```python
from build123d import *

# Parameters (mm, degrees)
F0_W     = 10
F0_H     = 40
F1_DEPTH = 180
F2_R     = 7
F3_DEPTH = 10.001
F4_W     = 40
F4_H     = 40
F4_R     = 7
F5_DEPTH = 10


with BuildPart() as f1:
    # F0 (on Right) → F1 (new body)
    with BuildSketch(Plane.YZ):
        Rectangle(F0_W, F0_H)
    extrude(amount=-F1_DEPTH)

    # F2 (on face) → F3 (cut, through all)
    with BuildSketch(Plane.XZ.offset(5)):
        with Locations((-160, 0)):
            Circle(F2_R)
        with Locations((-20, 0)):
            Circle(F2_R)
    extrude(amount=-F3_DEPTH, mode=Mode.SUBTRACT)

    # F4 (on face) → F5 (join)
    with BuildSketch(Plane.XZ.offset(5)):
        with Locations((-20, 0)):
            Rectangle(F4_W, F4_H)
        with Locations((-20, 0)):
            Circle(F4_R, mode=Mode.SUBTRACT)
    extrude(amount=F5_DEPTH)


solid = f1.part
```
Check sheet for the modelled part. Datum: model origin and axes. Units: mm. A direction names the side the tool comes from. Coordinates: 2 decimals unless noted, no trailing zeros. Loops run counter-clockwise (first coordinate to the right, second up) from the corner with the lowest first, then second, coordinate; pieces in that order, holes last.
1) Access from +Z, -Z, +X, -X, +Y, -Y to the whole of each face (thin tool, end or side, straight path). Record for faces 1 (the face through (-40, -10, 0)), 2 (the face through (-89, 5, 0)).
2) Gauge pin test, flat ends, axial feed: pin 1 (12 mm diameter, centred on x = -142.5, z = 2.5, fed in from -Y); pin 2 (1.5 mm diameter, centred on x = -88, y = -7, fed in from +Z); pin 3 (8 mm diameter, centred on y = -11.5, z = 0, fed in from -X). Record the tip position at first contact, or that the pin passes through.
3) Sectioned sample at C-C (y = -1). Record the boundary of the cut face in (x, z), and give its area (3 significant figures).
4) Sectioned sample at A-A (x = -160). Record the boundary of the cut face in (y, z).
5) Material ranges on probe 1 along X at (y, z) = (-1.5, -0.5); probe 2 along Z at (x, y) = (-20, -3); probe 3 along X at (y, z) = (-1.5, -5), recorded low to high.
6) Release check for a two-part mould opening along Z. For faces 3 (the face through (-71, -3, 20)), 4 (the face through (-71, -3, -20)), 5 (the face through (0, -5, 0)), 6 (the face through (-153.534, -0.07, -2.681)) record: released by +Z, released by -Z, zero draft, split by the parting line, or undercut.
7) Sectioned sample at B-B (z = 0). Record the boundary of the cut face in (x, y).
8) Sectioned sample at D-D (z = -13.5). Record the boundary of the cut face in (x, y).
Check sheet entries:
1. face 1: +Z, -Z, -X, -Y
1. face 2: +Z, -Z, +X, -X, +Y
2. pin 1: stops at y = -5
2. pin 2: passes through
2. pin 3: stops at x = -40
3. outline: (-180, -20) - (0, -20) - (0, 20) - (-180, 20) - close; hole circle Ø14 at (-160, 0); hole circle Ø14 at (-20, 0)
3. area: 6,890 mm2
4. outline: (-5, -20) - (5, -20) - (5, -7) - (-5, -7) - close; (-5, 7) - (5, 7) - (5, 20) - (-5, 20) - close
5. probe 1: x = -180 to -166.98, -153.02 to -26.98, -13.02 to 0
5. probe 2: z = -20 to -7, 7 to 20
5. probe 3: x = -180 to -164.9, -155.1 to -24.9, -15.1 to 0
6. face 3: released by +Z
6. face 4: released by -Z
6. face 5: zero draft
6. face 6: undercut
7. outline: (-180, -5) - (-167, -5) - (-167, 5) - (-180, 5) - close; (-153, -5) - (-40, -5) - (-40, -15) - (-27, -15) - (-27, 5) - (-153, 5) - close; (-13, -15) - (0, -15) - (0, 5) - (-13, 5) - close
8. outline: (-180, -5) - (-40, -5) - (-40, -15) - (0, -15) - (0, 5) - (-180, 5) - close
